```python
from build123d import *

# Parameters (mm, degrees)
F0_W     = 80
F0_H     = 50
F1_DEPTH = 40
F3_DEPTH = 30
F4_R     = 10
F5_DEPTH = 30
F7_DEPTH = 50
F8_R     = 15
F9_DEPTH = 50


with BuildPart() as f1:
    # F0 (on Top) → F1 (new body)
    with BuildSketch(Plane.XY):
        Rectangle(F0_W, F0_H)
    extrude(amount=F1_DEPTH)

    # F2 (on face) → F3 (join)
    with BuildSketch(Plane.XY.offset(40)):
        Polygon((0, 20.207259), (-17.5, -10.10363), (17.5, -10.10363), align=None)
    extrude(amount=F3_DEPTH)

    # F4 (on face) → F5 (cut)
    with BuildSketch(Plane.XY.offset(70)):
        Circle(F4_R)
    extrude(amount=-F5_DEPTH, mode=Mode.SUBTRACT)

    # F6 (on face) → F7 (join)
    with BuildSketch(Plane(origin=(0, 0, 0), x_dir=(1, 0, 0), z_dir=(0, 0, -1))):
        Polygon((-9.5, 10.322864), (-24.5, 10.322864), (-29.135255, -3.942983), (-17, -12.759762), (-4.864745, -3.942983), align=None)
    extrude(amount=F7_DEPTH)

    # F8 (on face) → F9 (join)
    with BuildSketch(Plane(origin=(0, 0, 0), x_dir=(1, 0, 0), z_dir=(0, 0, -1))):
        with Locations((22, 0)):
            Circle(F8_R)
    extrude(amount=F9_DEPTH)


solid = f1.part
```
Here's how the part is built. I have some questions about the finished solid (model axes, mm). A direction names the side the tool comes from. Coordinates: 2 decimals unless noted, no trailing zeros. Order: outer loops, then holes, each group sorted by start corner. A loop starts at its lowest first (then second) coordinate and runs counter-clockwise, first axis right, second up. Notation, with made-up numbers: (-16, 25) - (29, 25) arc R5 ccw to (29, 30) - close; hole circle Ø8 at (81, 1.25). An arc over 180 degrees is marked (long way). One line per question, with ' | ' between items.
(1) For faces 4 (the flat face through (-23.15, 8.29, -24.65)), 5 (the flat face through (4, -10.104, 55)), 6 (the flat face through (-26.785, -3.29, -24.65)), which set-ups out of +Z, -Z, +X, -X, +Y, -Y let a thin tool reach every point of the face, with its end or its side?
Report:
face 4: -Z, -X, +Y | face 5: +Z, +X, -X, -Y | face 6: -Z, -X, -Y
(2) Suppose I cut it at B-B on z = -11. List the corners of the cut face in (x, y) for me, and give its area (3 significant figures).
Report:
outline: (-29.14, 3.94) - (-24.5, -10.32) - (-9.5, -10.32) - (-4.86, 3.94) - (-17, 12.76) - close; circle Ø30 at (22, 0) | area: 1,090 mm2
(3) Suppose I cut it at D-D on x = 12. List the corners of the cut face in (y, z) for me, and give its area (3 significant figures).
Report:
outline: (-25, 0) - (-11.18, 0) - (-11.18, -50) - (11.18, -50) - (11.18, 0) - (25, 0) - (25, 40) - (-0.58, 40) - (-0.58, 70) - (-10.1, 70) - (-10.1, 40) - (-25, 40) - close | area: 3,400 mm2
(4) Suppose I cut it at C-C on y = 17. List the corners of the cut face in (x, z) for me.
Report:
outline: (-40, 0) - (40, 0) - (40, 40) - (1.85, 40) - (1.85, 70) - (-1.85, 70) - (-1.85, 40) - (-40, 40) - close
(5) Will these pins go through, and if not, where does the flat tip stop? pin 1 (4 mm diameter, centred on x = -12, y = 7, fed in from +Z); pin 2 (10 mm diameter, centred on x = 17.5, z = -15.5, fed in from +Y); pin 3 (16.5 mm diameter, centred on x = -20.5, z = -25.5, fed in from -Y).
Report:
pin 1: stops at z = 40 | pin 2: stops at y = 15 | pin 3: stops at y = -10.32
(6) If I drill on L1, parallel to Z at x = 26, y = 11; L2, parallel to Z at x = 7.5, y = -10; L3, parallel to Y at x = 2, z = 58, over which ranges is the centre line in solid material (lowest first)?
Report:
L1: z = -50 to 40 | L2: z = 0 to 70 | L3: y = -10.1 to -9.8, 9.8 to 16.74
(7) If we mould it in two halves opening along Y, with no side actions, what happens to faces 1 (the flat face through (-6.7, 8.6, 54.8)), 2 (the flat face through (-17, 1, -50)), 3 (the flat face through (0, 0, 40))? For each: pulls with the +Y half, pulls with the -Y half, needs draft (parallel to the pull), parting line crosses it, or undercut.
Report:
face 1: pulls with the +Y half | face 2: needs draft | face 3: undercut
(8) Suppose I cut it at A-A on x = 22. List the corners of the cut face in (y, z) for me, and give its area (3 significant figures).
Report:
outline: (-25, 0) - (-15, 0) - (-15, -50) - (15, -50) - (15, 0) - (25, 0) - (25, 40) - (-25, 40) - close | area: 3,500 mm2
